Work out the finished part from the listing and answer in its coordinate system (mm). A direction names the side the tool comes from. Coordinates: 2 decimals unless noted, no trailing zeros. Order: outer loops, then holes, each group sorted by start corner. A loop starts at its lowest first (then second) coordinate and runs counter-clockwise, first axis right, second up. Notation, with made-up numbers: (78, 11) -> (120, 11) arc R18 cw to (120, 25) -> close; hole circle Ø7 at (70, 85.5). An arc over 180 degrees is marked (long way). Use one line per item in the form item = value.
from build123d import *

# Parameters (mm, degrees)
SKETCH1_W           = 35
SKETCH1_H           = 35
BOSS_EXTRUDE1_DEPTH = 10
SKETCH2_W           = 32
SKETCH2_H           = 32
CUT_EXTRUDE1_DEPTH  = 9
BOSS_EXTRUDE2_DEPTH = 3
SKETCH5_R           = 1.5
CUT_EXTRUDE2_DEPTH  = 51.309044912


with BuildPart() as part:
    # Sketch1 → Boss-Extrude1 (new body)
    with BuildSketch(Plane.XY):
        with Locations((17.5, -17.5)):
            Rectangle(SKETCH1_W, SKETCH1_H)
    extrude(amount=BOSS_EXTRUDE1_DEPTH)

    # Sketch2 → Cut-Extrude1 (cut)
    with BuildSketch(Plane.XY.offset(10)):
        with Locations((17.5, -17.5)):
            Rectangle(SKETCH2_W, SKETCH2_H)
    extrude(amount=-CUT_EXTRUDE1_DEPTH, mode=Mode.SUBTRACT)

    # Sketch3 → Boss-Extrude2 (add)
    with BuildSketch(Plane.XY.offset(1)):
        Polygon((3.1, -3.1), (3.1, -9.6), (4.6, -9.6), (4.6, -4.6), (9.6, -4.6), (9.6, -3.1), align=None)
        Polygon((4.6, -30.4), (9.6, -30.4), (9.6, -31.9), (3.1, -31.9), (3.1, -25.4), (4.6, -25.4), align=None)
        Polygon((30.4, -30.4), (30.4, -25.4), (31.9, -25.4), (31.9, -31.9), (25.4, -31.9), (25.4, -30.4), align=None)
        Polygon((30.4, -4.6), (25.4, -4.6), (25.4, -3.1), (31.9, -3.1), (31.9, -9.6), (30.4, -9.6), align=None)
    extrude(amount=BOSS_EXTRUDE2_DEPTH)

    # Sketch5 → Cut-Extrude2 (cut, through all)
    with BuildSketch(Plane.XY.offset(1)):
        with Locations((7.34, -7.34)):
            Circle(SKETCH5_R)
        with Locations((7.34, -27.66)):
            Circle(SKETCH5_R)
        with Locations((27.66, -27.66)):
            Circle(SKETCH5_R)
        with Locations((27.66, -7.34)):
            Circle(SKETCH5_R)
    extrude(amount=-CUT_EXTRUDE2_DEPTH, mode=Mode.SUBTRACT)


solid = part.part
(1) Straight lines are drawn through the part: line 1 along Y through (x, z) = (15, 8.5); line 2 along Y through (x, z) = (7.34, 0.3); line 3 along X through (y, z) = (-20, 8). For each, find the intervals that lie inside material, in ascending order.
Data:
line_1 = -35 to -33.5, -1.5 to 0
line_2 = -35 to -29.16, -26.16 to -8.84, -5.84 to 0
line_3 = 0 to 1.5, 33.5 to 35
(2) Section A-A on z = 1.5 is taken. Count the separate pieces of the cut face and the enclosed holes in it, plus the area to 3 significant figures.
Data:
separate_pieces = 5
enclosed_holes = 1
area = 270 mm²
(3) Section B-B on y = -27.66 is taken. Write down the section's boundary in (x, z).
Data:
outline = (0, 0) -> (5.84, 0) -> (5.84, 1) -> (4.6, 1) -> (4.6, 4) -> (3.1, 4) -> (3.1, 1) -> (1.5, 1) -> (1.5, 10) -> (0, 10) -> close; (8.84, 0) -> (26.16, 0) -> (26.16, 1) -> (8.84, 1) -> close; (29.16, 0) -> (35, 0) -> (35, 10) -> (33.5, 10) -> (33.5, 1) -> (31.9, 1) -> (31.9, 4) -> (30.4, 4) -> (30.4, 1) -> (29.16, 1) -> close
(4) Which of the six approach directions +Z, -Z, +X, -X, +Y, -Y give full straight-line access (tool end or side, diameter ignored) to faces 4 (the cylindrical face through (29.09, -6.89, 0.51)), 5 (the flat face through (30.4, -28, 2))?
Data:
face_4 = +Z, -Z
face_5 = +Z
(5) Each of these flat-tipped pins is pushed along its axis until it touches: P1, Ø5, axis at x = 6.5, y = -5.5, coming from the +Z side; P2, Ø4, axis at x = 7.34, y = -7.34, coming from the +Z side. Where does it stop, or does it pass through?
Data:
P1 = 4
P2 = 1
(6) Section D-D on x = 15.5 is taken. Write down the section's boundary in (y, z), plus the area to 3 significant figures.
Data:
outline = (-35, 0) -> (0, 0) -> (0, 10) -> (-1.5, 10) -> (-1.5, 1) -> (-33.5, 1) -> (-33.5, 10) -> (-35, 10) -> close
area = 62.0 mm²
(7) The mould has two halves that part along X. Classify faces 1 (the flat face through (0, -18, 5)), 2 (the flat face through (16, -34, 10)), 3 (the flat face through (17, -33.5, 6)): released by +X, released by -X, zero draft, split by the parting line, or undercut.
Data:
face_1 = released by -X
face_2 = zero draft
face_3 = undercut
(8) Section C-C on x = 7.34 is taken. Write down the section's boundary in (y, z).
Data:
outline = (-35, 0) -> (-29.16, 0) -> (-29.16, 1) -> (-30.4, 1) -> (-30.4, 4) -> (-31.9, 4) -> (-31.9, 1) -> (-33.5, 1) -> (-33.5, 10) -> (-35, 10) -> close; (-26.16, 0) -> (-8.84, 0) -> (-8.84, 1) -> (-26.16, 1) -> close; (-5.84, 0) -> (0, 0) -> (0, 10) -> (-1.5, 10) -> (-1.5, 1) -> (-3.1, 1) -> (-3.1, 4) -> (-4.6, 4) -> (-4.6, 1) -> (-5.84, 1) -> close
